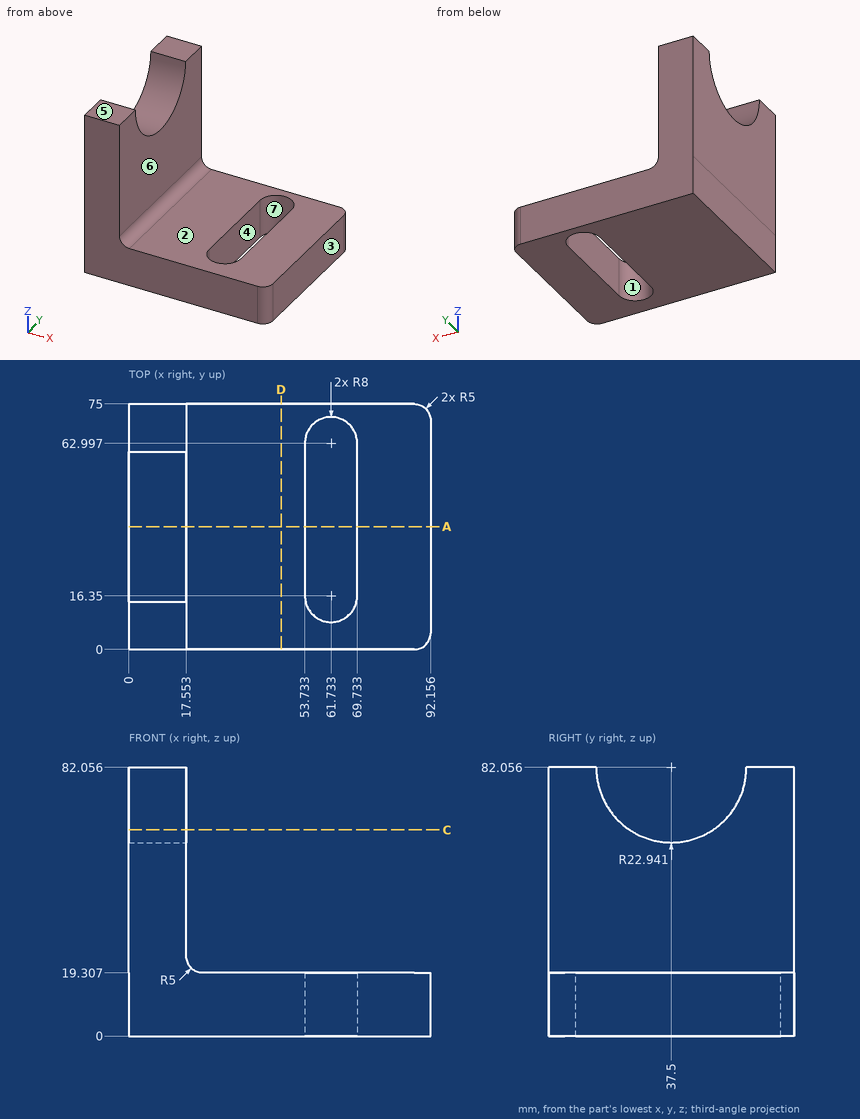
Geometry check sheet. Reference: drawing and pictorial views, mm from the part's lowest x, y, z. A direction names the side the tool comes from. Coordinates: 2 decimals unless noted, no trailing zeros. Order: outer loops, then holes, each group sorted by start corner. A loop starts at its lowest first (then second) coordinate and runs counter-clockwise, first axis right, second up. Notation, with made-up numbers: (-10.75, -2) -> (2.25, -2) arc R18 ccw to (2.25, 23) -> close; hole circle Ø1 at (-33.75, 60.5). An arc over 180 degrees is marked (long way). Use CSV: the item, a comma, the result in double quotes. Start each with the question number.
Q1. Draft check along X on the marked faces 4, 5, 6 and 7. Enter one of: +X half, -X half, draft (parallel to the pull), parting line (faces both ways), or undercut.
Q2. Section check A-A, the plane y = 37.5. Record the cut outline in (x, z) (1 decimal).
Q3. Thickness scan on line 1 along Z through (x, y) = (32.5, 54); line 2 along X through (y, z) = (20, 38); line 3 along Y through (x, z) = (62.5, 14.5). Record the ranges inside material, lowest first.
Q4. Depth check by flat-ended pin: P1, Ø10, axis at x = 62.5, y = 42, coming from the -Z side; P2, Ø2, axis at y = 33, z = 29.5, coming from the +X side; P3, Ø12, axis at x = 73.5, y = 40.5, coming from the +Z side. Enter the tip coordinate at first touch or a pass-through.
Q5. Tool access check on the marked faces 1, 2 and 3. Record the directions out of +Z, -Z, +X, -X, +Y, -Y that give a thin tool (end or side, any length) a straight path to the whole face; none if there is none.
Q6. Section check D-D, the plane x = 46.5. Record the cut outline in (y, z).
Q7. Section check C-C, the plane z = 63. Record the cut outline in (x, y), and give its area (3 significant figures).
Returned:
1,face 4,"undercut"
1,face 5,"draft"
1,face 6,"+X half"
1,face 7,"undercut"
2,outline,"(0, 0) -> (53.7, 0) -> (53.7, 19.3) -> (22.6, 19.3) arc R5 cw to (17.6, 24.3) -> (17.6, 59.1) -> (0, 59.1) -> close; (69.7, 0) -> (92.2, 0) -> (92.2, 19.3) -> (69.7, 19.3) -> close"
3,line 1,"z = 0 to 19.31"
3,line 2,"x = 0 to 17.55"
3,line 3,"y = 0 to 8.39, 70.96 to 75"
4,P1,"passes through"
4,P2,"stops at x = 17.55"
4,P3,"stops at z = 19.31"
5,face 1,"+Z, -Z"
5,face 2,"+Z, +X, +Y, -Y"
5,face 3,"+Z, -Z, +X, +Y, -Y"
6,outline,"(0, 0) -> (75, 0) -> (75, 19.31) -> (0, 19.31) -> close"
7,outline,"(0, 0) -> (17.55, 0) -> (17.55, 24.73) -> (0, 24.73) -> close; (0, 50.27) -> (17.55, 50.27) -> (17.55, 75) -> (0, 75) -> close"
7,area,"868 mm^2"
